For this review, take the finished solid that the model builds, in its own axes (mm). A direction names the side the tool comes from. Give positions to 0.01 mm unless a question says otherwise; leave off trailing zeros. Loops run counter-clockwise (first coordinate to the right, second up) from the corner with the lowest first, then second, coordinate; pieces in that order, holes last.
```python
from build123d import *

# Parameters (mm, degrees)
ESQUISSE1_W             = 146
ESQUISSE1_H             = 190
BOSS_EXTRU_1_DEPTH      = 5
ESQUISSE15_W            = 15
ESQUISSE15_H            = 20
BOSS_EXTRU_7_DEPTH      = 16
ESQUISSE16_W            = 15
ESQUISSE16_H            = 20
BOSS_EXTRU_8_DEPTH      = 16
ESQUISSE17_W            = 35
ESQUISSE17_H            = 35
ENL_V_MAT_EXTRU_1_DEPTH = 5


with BuildPart() as part:
    # Esquisse1 → Boss.-Extru.1 (new body)
    with BuildSketch(Plane.XY):
        with Locations((-35.228613981, 18.194490743)):
            Rectangle(ESQUISSE1_W, ESQUISSE1_H)
    extrude(amount=BOSS_EXTRU_1_DEPTH)

    # Esquisse15 → Boss.-Extru.7 (add)
    with BuildSketch(Plane.XY.offset(5)):
        with Locations((-100.228613981, -61.705509257)):
            Rectangle(ESQUISSE15_W, ESQUISSE15_H)
    extrude(amount=BOSS_EXTRU_7_DEPTH)

    # Esquisse16 → Boss.-Extru.8 (add)
    with BuildSketch(Plane.XY.offset(5)):
        with Locations((-100.228613981, 98.094490743)):
            Rectangle(ESQUISSE16_W, ESQUISSE16_H)
    extrude(amount=BOSS_EXTRU_8_DEPTH)

    # Esquisse17 → Enlèv. mat.-Extru.1 (cut)
    with BuildSketch(Plane.XY.offset(5)):
        with Locations((-35.228613981, 18.194490743)):
            Rectangle(ESQUISSE17_W, ESQUISSE17_H)
    extrude(amount=-ENL_V_MAT_EXTRU_1_DEPTH, mode=Mode.SUBTRACT)


solid = part.part
```
Item 1: Take a section at A-A on y = 25.5. Give the boundary of the cut face in (x, z), and give its area (3 significant figures).
Answer:
outline: (-108.23, 0) - (-52.73, 0) - (-52.73, 5) - (-108.23, 5) - close; (-17.73, 0) - (37.77, 0) - (37.77, 5) - (-17.73, 5) - close
area: 555 mm2
Item 2: For L1, parallel to Y at x = -96, z = 9.25; L2, parallel to Y at x = -23.5, z = 1.75; L3, parallel to X at y = 27.5, z = 1, list the stretches that pass through material, from the lowest coordinate up.
Answer:
L1: y = -71.71 to -51.71, 88.09 to 108.09
L2: y = -76.81 to 0.69, 35.69 to 113.19
L3: x = -108.23 to -52.73, -17.73 to 37.77
Item 3: Take a section at B-B on z = 13.5. Give the boundary of the cut face in (x, y).
Answer:
outline: (-107.73, -71.71) - (-92.73, -71.71) - (-92.73, -51.71) - (-107.73, -51.71) - close; (-107.73, 88.09) - (-92.73, 88.09) - (-92.73, 108.09) - (-107.73, 108.09) - close
Item 4: Tool access review of faces 1 (the flat face through (-92.729, -62, 13)), 2 (the flat face through (-107.729, -62, 13)), 3 (the flat face through (-35, 0.694, 3)): name each direction out of +Z, -Z, +X, -X, +Y, -Y from which nothing blocks a thin tool from reaching the whole face with its end or side.
Answer:
face 1: +Z, +X, +Y, -Y
face 2: +Z, -X, +Y, -Y
face 3: +Z, -Z
Item 5: Take a section at D-D on y = 98. Give the boundary of the cut face in (x, z), and give its area (3 significant figures).
Answer:
outline: (-108.23, 0) - (37.77, 0) - (37.77, 5) - (-92.73, 5) - (-92.73, 21) - (-107.73, 21) - (-107.73, 5) - (-108.23, 5) - close
area: 970 mm2
Item 6: Clearance check with flat-ended pins moving along their axes: pin 1 Ø3 at (x, y) = (-71, 7) entering from +Z; pin 2 Ø4.5 at (x, z) = (-97, 16) entering from -Y; pin 3 Ø5 at (y, z) = (-64, 15.5) entering from -X. State where each tip first meets the part, or that it passes through.
Answer:
pin 1: stops at z = 5
pin 2: stops at y = -71.71
pin 3: stops at x = -107.73
Item 7: The part is to be moulded in two halves that separate along X. For faces 4 (the flat face through (-17.729, 18, 3)), 5 (the flat face through (-92.729, 98, 13)), 6 (the flat face through (-107.729, 98, 13)), 7 (the flat face through (-36, 113.194, 2)), say which applies: released by +X, released by -X, zero draft, split by the parting line, or undercut.
Answer:
face 4: undercut
face 5: released by +X
face 6: released by -X
face 7: zero draft
Item 8: Take a section at C-C on z = 2.25. Give the boundary of the cut face in (x, y).
Answer:
outline: (-108.23, -76.81) - (37.77, -76.81) - (37.77, 113.19) - (-108.23, 113.19) - close; hole (-52.73, 0.69) - (-17.73, 0.69) - (-17.73, 35.69) - (-52.73, 35.69) - close
